Check sheet for the modelled part. Datum: model origin and axes. Units: mm. A direction names the side the tool comes from. Give positions to 0.01 mm unless a question says otherwise; leave off trailing zeros. Write each loop counter-clockwise with the first axis right and the second up, starting at its lowest first coordinate (ties: lowest second). Pieces come first, ordered by that corner, then holes. Notation, with made-up numbers: (-18.75, 56) -> (32.25, 56) arc R10 ccw to (32.25, 60) -> close; hole circle Ø2 at (44, 40). An arc over 180 degrees is marked (long way). Return JSON: item names as keys, results as strings.
from build123d import *

# Parameters (mm, degrees)
SKETCH_1_R          = 15
SKETCH_1_R_2        = 1.75
EXTRUDE_1_DEPTH     = 14
SKETCH_2_R          = 5.15
CUT_EXTRUDE_1_DEPTH = 4
FILLET_1_R          = 2
FILLET_2_R          = 7


with BuildPart() as part:
    # Эскиз1 → Бобышка-Вытянуть1 (new body)
    with BuildSketch(Plane.XY):
        Circle(SKETCH_1_R)
        Circle(SKETCH_1_R_2, mode=Mode.SUBTRACT)
    extrude(amount=EXTRUDE_1_DEPTH)

    # Эскиз2 → Вырез-Вытянуть1 (cut)
    with BuildSketch(Plane.XY.offset(14)):
        Circle(SKETCH_2_R)
    extrude(amount=-CUT_EXTRUDE_1_DEPTH, mode=Mode.SUBTRACT)

    # Скругление1
    fillet_1_edges = [part.edges().sort_by_distance(p)[0] for p in [
        (-15, 0, 14),
    ]]
    fillet(fillet_1_edges, radius=FILLET_1_R)

    # Скругление2
    fillet_2_edges = [part.edges().sort_by_distance(p)[0] for p in [
        (-15, 0, 0),
    ]]
    fillet(fillet_2_edges, radius=FILLET_2_R)


solid = part.part
(1) Depth check by flat-ended pin: pin 1 Ø8 at (x, z) = (-4, 5) entering from -Y; pin 2 Ø8 at (y, z) = (5.5, 11) entering from +X; pin 3 Ø3 at (x, y) = (0, 0) entering from -Z; pin 4 Ø2 at (x, z) = (9.5, 7.5) entering from -Y. Enter the tip coordinate at first touch or a pass-through.
Reply:
{"pin 1": "y = -14.99", "pin 2": "x = 14.92", "pin 3": "through", "pin 4": "y = -12.36"}
(2) Release check for a two-part mould opening along X. For faces 3 (the cylindrical face through (1.617, -0.67, 4.93)), 4 (the flat face through (6, 0, 14)), 5 (the cylindrical face through (-14.985, 0.66, 9.465)) record: pulls with the +X half, pulls with the -X half, needs draft (parallel to the pull), parting line crosses it, or undercut.
Reply:
{"face 3": "undercut", "face 4": "needs draft", "face 5": "parting line crosses it"}
(3) Cross-section at C-C on z = 7.5. Enter the section's corners in (x, y).
Reply:
{"outline": "circle Ø30 at (0, 0); hole circle Ø3.5 at (0, 0)"}
(4) Set-up check for faces 1 (the flat face through (0, 2, 0)), 2 (the cylindrical face through (4.91, 1.55, 12.03)): record each of +Z, -Z, +X, -X, +Y, -Y from which the full face is reachable in a straight line by a thin tool's end or side.
Reply:
{"face 1": "-Z, +X, -X, +Y, -Y", "face 2": "+Z"}
(5) Thickness scan on L1, parallel to Y at x = 0, z = 11; L2, parallel to Y at x = 0, z = 7.75; L3, parallel to Z at x = -1, y = 4. Record the ranges inside material, lowest first.
Reply:
{"L1": "-15 to -5.15, 5.15 to 15", "L2": "-15 to -1.75, 1.75 to 15", "L3": "0 to 10"}
(6) Cross-section at A-A on y = 0. Enter the section's corners in (x, z), then the cut area to 3 significant figures.
Reply:
{"outline": "(-15, 7) arc R7 ccw to (-8, 0) -> (-1.75, 0) -> (-1.75, 10) -> (-5.15, 10) -> (-5.15, 14) -> (-13, 14) arc R2 ccw to (-15, 12) -> close; (1.75, 0) -> (8, 0) arc R7 ccw to (15, 7) -> (15, 12) arc R2 ccw to (13, 14) -> (5.15, 14) -> (5.15, 10) -> (1.75, 10) -> close", "area": "321 mm^2"}
(7) Cross-section at D-D on z = 10.5. Enter the section's corners in (x, y).
Reply:
{"outline": "circle Ø30 at (0, 0); hole circle Ø10.3 at (0, 0)"}
